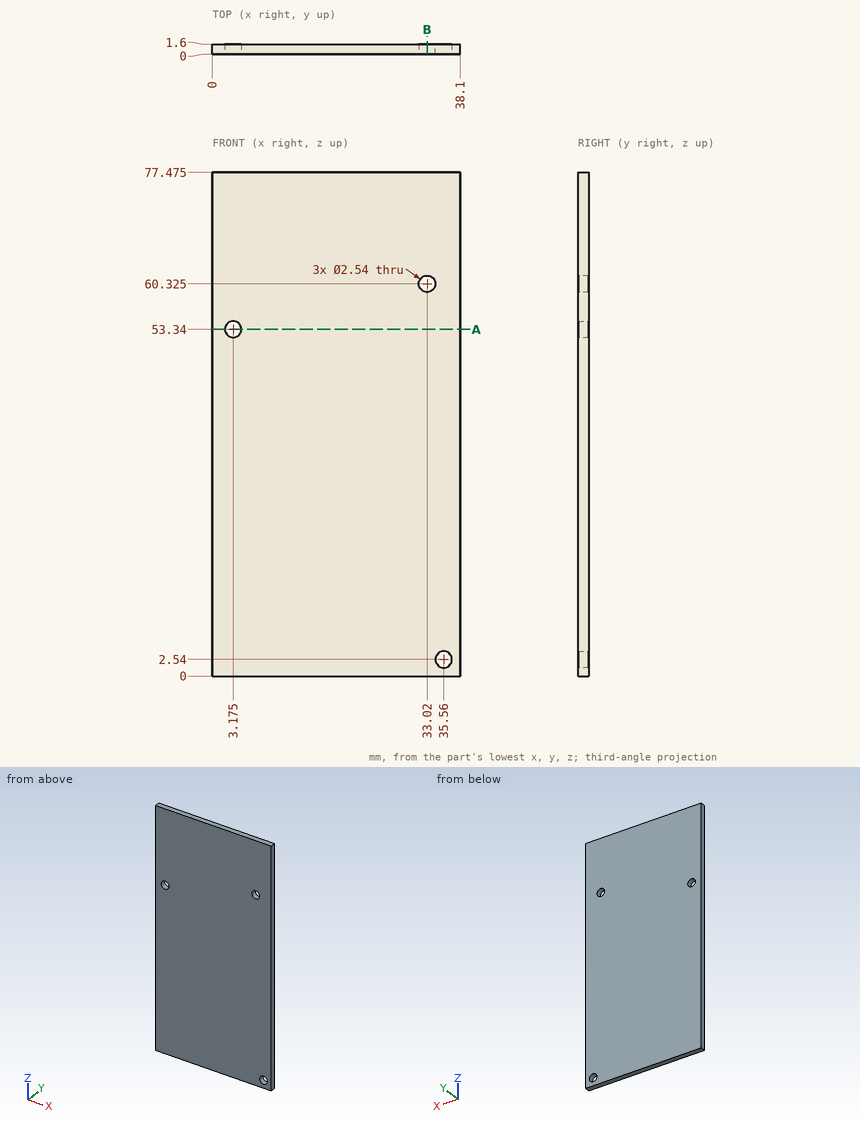
Source: three-view drawing plus pictorial views. Frame: mm from the lowest corner of the part. Give positions to 0.01 mm unless a question says otherwise; leave off trailing zeros. Write each loop counter-clockwise with the first axis right and the second up, starting at its lowest first coordinate (ties: lowest second). Pieces come first, ordered by that corner, then holes. Notation, with made-up numbers: (-39.5, -25.5) - (-23.5, -25.5) arc R19 ccw to (-23.5, -21.5) - close; hole circle Ø2 at (48.5, 6). An arc over 180 degrees is marked (long way). Write item = value, one per line. Start each with the question number.
Q1. Cut plane B-B, the plane x = 33.02. Return loops of the section in (y, z) (3 decimals), then the cut area to 3 significant figures.
Q2. Material intervals for probe 1 along Z at (x, y) = (33.02, 0.35) (3 decimals); probe 2 along Z at (x, y) = (35.56, 0.4) (3 decimals); probe 3 along X at (y, z) = (0.5, 53.34) (3 decimals), sorted ascending.
Q3. Cut plane A-A, the plane z = 53.34. Return loops of the section in (x, y) (3 decimals), then the cut area to 3 significant figures.
Computed values:
q1.outline = (0, 0) - (1.6, 0) - (1.6, 59.055) - (0, 59.055) - close; (0, 61.595) - (1.6, 61.595) - (1.6, 77.475) - (0, 77.475) - close
q1.area = 120 mm²
q2.probe_1 = 0 to 59.055, 61.595 to 77.475
q2.probe_2 = 0 to 1.27, 3.81 to 77.475
q2.probe_3 = 0 to 1.905, 4.445 to 38.1
q3.outline = (0, 0) - (1.905, 0) - (1.905, 1.6) - (0, 1.6) - close; (4.445, 0) - (38.1, 0) - (38.1, 1.6) - (4.445, 1.6) - close
q3.area = 56.9 mm²
